from build123d import *

# Parameters (mm, degrees)
BOSS_EXTRUDE1_DEPTH = 13
SKETCH8_R           = 1.65
CUT_EXTRUDE4_DEPTH  = 14
SKETCH6_R           = 6
BOSS_EXTRUDE2_DEPTH = 10
SKETCH4_R           = 2.15
CUT_EXTRUDE3_DEPTH  = 20


with BuildPart() as part:
    # Sketch2 → Boss-Extrude1 (new body)
    with BuildSketch(Plane.XY):
        with BuildLine():
            Line((7, -5), (-7, -5))
            ThreePointArc((-7, -5), (-10.090169944, 0), (-7, 5))
            Line((-7, 5), (7, 5))
            ThreePointArc((7, 5), (10.090169944, 0), (7, -5))
        make_face()
    extrude(amount=BOSS_EXTRUDE1_DEPTH)

    # Sketch8 → Cut-Extrude4 (cut, through all)
    with BuildSketch(Plane(origin=(0, 0, 0), x_dir=(-1, 0, 0), z_dir=(0, 0, -1))):
        with Locations((-5.05, 0)):
            Circle(SKETCH8_R)
        with Locations((5.05, 0)):
            Circle(SKETCH8_R)
    extrude(amount=-CUT_EXTRUDE4_DEPTH, mode=Mode.SUBTRACT)

    # Sketch6 → Boss-Extrude2 (add)
    with BuildSketch(Plane.XZ.offset(5)):
        with Locations(Location((0, 6.5, 0), (0, 0, 180))):  # turned: the seam where the file's is
            Circle(SKETCH6_R)
    extrude(amount=BOSS_EXTRUDE2_DEPTH)

    # Sketch4 → Cut-Extrude3 (cut)
    with BuildSketch(Plane(origin=(0, 5, 0), x_dir=(1, 0, 0), z_dir=(0, 1, 0))):
        with Locations(Location((0, -6.5, 0), (0, 0, 180))):  # turned: the seam where the file's is
            Circle(SKETCH4_R)
    extrude(amount=-CUT_EXTRUDE3_DEPTH, mode=Mode.SUBTRACT)


solid = part.part
Geometry: final body of the model. Coordinates: model frame, mm. A direction names the side the tool comes from. Coordinates: 2 decimals unless noted, no trailing zeros. Loops run counter-clockwise (first coordinate to the right, second up) from the corner with the lowest first, then second, coordinate; pieces in that order, holes last. Notation, with made-up numbers: (-0.75, 6) - (38.25, 6) arc R33 ccw to (38.25, 41) - close; hole circle Ø4 at (-20.75, 69.25). An arc over 180 degrees is marked (long way). Put each result on its own line as item: value. Start each with the question number.
Q1. Pin query (flat end, axial travel): pin 1 Ø3 at (x, y) = (5.05, 0) entering from -Z; pin 2 Ø2 at (y, z) = (-10, 5) entering from +X; pin 3 Ø5 at (y, z) = (-3.5, 5.5) entering from +X. Return the tip coordinate at first contact, or that it passes through.
Q2. Cut plane D-D, the plane z = 2. Return loops of the section in (x, y).
Q3. Line query: line 1 (Y direction, x = -5.05, z = 9.5); line 2 (Z direction, x = 0, y = -9); line 3 (Z direction, x = 0, y = 4.25). Output: solid intervals per line, ascending.
Q4. Set-up query: faces 4 (the cylindrical face through (-2.769, -9.93, 11.823)), 5 (the flat face through (0, 0, 0)). Return all of +Z, -Z, +X, -X, +Y, -Y with unobstructed straight access to the full face (end or side cutting, diameter ignored); none if empty.
Q5. Cut plane A-A, the plane y = 0. Return loops of the section in (x, z).
Q6. Cut plane C-C, the plane x = 0.25. Return loops of the section in (y, z).
Q7. Cut plane B-B, the plane z = 6.5. Return loops of the section in (x, y), and give its area (3 significant figures).
Q8. Pull-direction query (X, two-part tool) for faces 1 (the flat face through (-5, -5, 2)), 2 (the cylindrical face through (6.36, -1, 6.41)), 3 (the cylindrical face through (10.09, 0.09, 6.41)); classes: released by +X, released by -X, zero draft, split by the parting line, or undercut.
Filled sheet:
1. pin 1: through
1. pin 2: x = 5.98
1. pin 3: x = 10
2. outline: (-7, -5) - (-3.97, -5) - (-3.97, -15) - (3.97, -15) - (3.97, -5) - (7, -5) arc R5.59 ccw to (7, 5) - (-7, 5) arc R5.59 ccw to start; hole circle Ø3.3 at (-5.05, 0); hole circle Ø3.3 at (5.05, 0)
3. line 1: -15 to -1.65, 1.65 to 5
3. line 2: 0.5 to 4.35, 8.65 to 12.5
3. line 3: 0 to 4.35, 8.65 to 13
4. face 4: -Y
4. face 5: -Z, +X, -X, +Y, -Y
5. outline: (-10.09, 0) - (-6.7, 0) - (-6.7, 13) - (-10.09, 13) - close; (-3.4, 0) - (3.4, 0) - (3.4, 13) - (-3.4, 13) - close; (6.7, 0) - (10.09, 0) - (10.09, 13) - (6.7, 13) - close; hole circle Ø4.3 at (0, 6.5)
6. outline: (-15, 0.51) - (-5, 0.51) - (-5, 0) - (5, 0) - (5, 4.36) - (-15, 4.36) - close; (-15, 8.64) - (5, 8.64) - (5, 13) - (-5, 13) - (-5, 12.49) - (-15, 12.49) - close
7. outline: (-7, -5) - (-6, -5) - (-6, -15) - (-2.15, -15) - (-2.15, 5) - (-7, 5) arc R5.59 ccw to start; (2.15, -15) - (6, -15) - (6, -5) - (7, -5) arc R5.59 ccw to (7, 5) - (2.15, 5) - close; hole circle Ø3.3 at (-5.05, 0); hole circle Ø3.3 at (5.05, 0)
7. area: 201 mm²
8. face 1: zero draft
8. face 2: undercut
8. face 3: released by +X
